Geometry: see drawing. Coordinates: mm, zero at the bounding-box minimum. A direction names the side the tool comes from. Round coordinates to 2 decimals unless told otherwise and drop trailing zeros. Order: outer loops, then holes, each group sorted by start corner. A loop starts at its lowest first (then second) coordinate and runs counter-clockwise, first axis right, second up. Notation, with made-up numbers: (18, -18) - (47, -18) arc R6 ccw to (47, -12) - close; hole circle Ø11 at (27, 74). An arc over 180 degrees is marked (long way). Put each result on its own line as item: value. Start each with the question number.
1) Line query: probe 1 along X at (y, z) = (67.5, 62); probe 2 along Z at (x, y) = (211.5, 119); probe 3 along Y at (x, z) = (14, 95.5). Output: solid intervals per line, ascending. Write a range as [from, to].
2) Section A-A on x = 303. Output: boundary loops of the cut face in (y, z).
3) Section B-B on y = 97. Output: boundary loops of the cut face in (x, z), then the cut area to 3 significant figures.
4) Access query for the marked faces 4 and 5. Directions: +Z, -Z, +X, -X, +Y, -Y. A direction counts if a zero-diameter tool reaches every point of the face in a straight line with its end or side. Return the directions, or none.
5) Contact query for a flat-ended pin moving along its axis: P1, Ø8, axis at x = 73, z = 289, coming from the +Y side. Output: stop coordinate, or through.
6) Mould query, pull axis X, two halves, no side actions, for the marked faces 1, 2 and 3. Classes: +X half, -X half, draft (parallel to the pull), parting line (faces both ways), or undercut.
7) Section C-C on z = 593. Output: boundary loops of the cut face in (x, y), then the cut area to 3 significant figures.
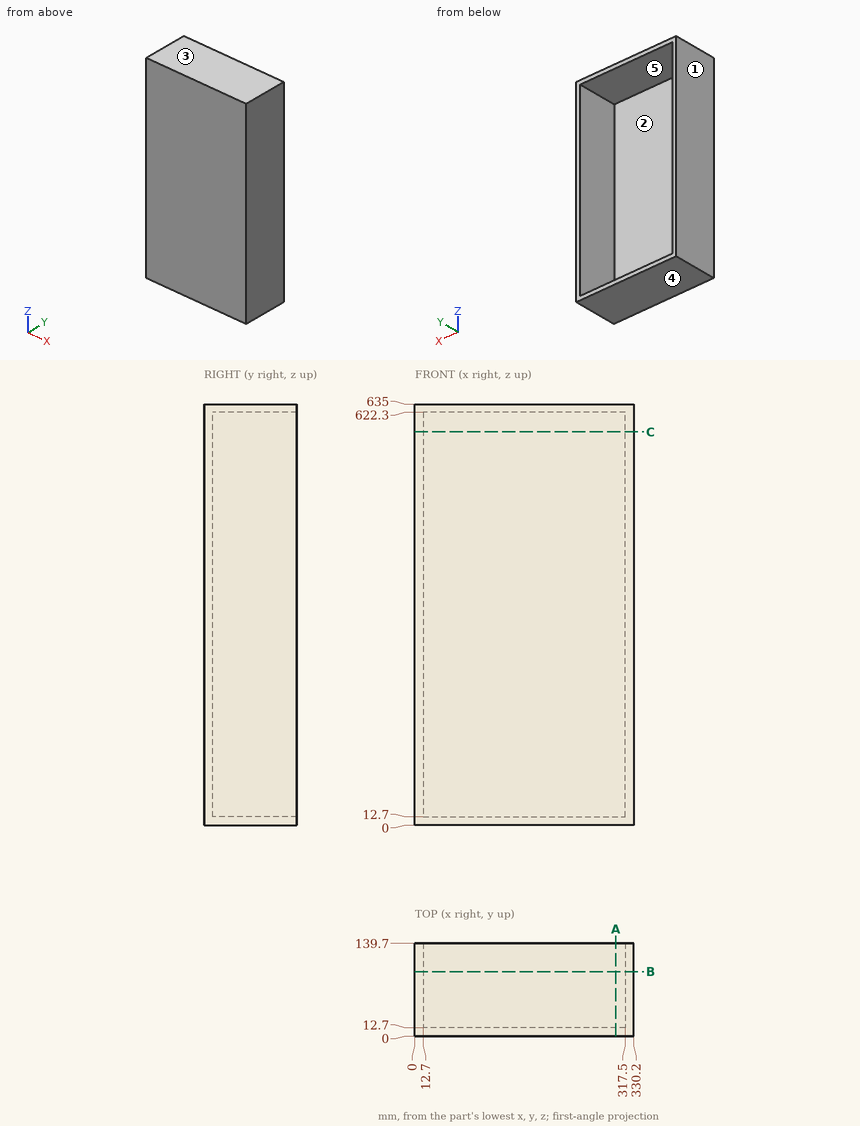
Answer sheet:
1. probe 1: [0, 12.7], [317.5, 330.2]
1. probe 2: [0, 12.7], [622.3, 635]
1. probe 3: [0, 12.7]
2. outline: (0, 0) - (139.7, 0) - (139.7, 12.7) - (12.7, 12.7) - (12.7, 622.3) - (139.7, 622.3) - (139.7, 635) - (0, 635) - close
3. outline: (0, 0) - (330.2, 0) - (330.2, 635) - (0, 635) - close; hole (12.7, 12.7) - (317.5, 12.7) - (317.5, 622.3) - (12.7, 622.3) - close
3. area: 23,900 mm^2
4. face 4: -Z, +X, -X, +Y, -Y
4. face 5: +Y
5. P1: y = 12.7
6. face 1: -X half
6. face 2: undercut
6. face 3: draft
7. outline: (0, 0) - (330.2, 0) - (330.2, 139.7) - (317.5, 139.7) - (317.5, 12.7) - (12.7, 12.7) - (12.7, 139.7) - (0, 139.7) - close
7. area: 7,420 mm^2
